from build123d import *

# Parameters (mm, degrees)
CROQUIS1_W              = 309
CROQUIS1_H              = 195
CROQUIS1_W_2            = 227
CROQUIS1_H_2            = 113
SALIENTE_EXTRUIR1_DEPTH = 15
CROQUIS2_R              = 2.75
CORTAR_EXTRUIR1_DEPTH   = 7.5


with BuildPart() as part:
    # Croquis1 → Saliente-Extruir1 (new body)
    with BuildSketch(Plane.YZ):
        with Locations((154.5, 97.5)):
            Rectangle(CROQUIS1_W, CROQUIS1_H)
        with Locations((154.5, 97.5)):
            Rectangle(CROQUIS1_W_2, CROQUIS1_H_2, mode=Mode.SUBTRACT)
    extrude(amount=SALIENTE_EXTRUIR1_DEPTH)

    # Croquis2 → Cortar-Extruir1 (cut)
    with BuildSketch(Plane.YZ.offset(15)):
        with BuildLine():
            ThreePointArc((66.75, 41), (64, 43.75), (61.25, 41))
            Line((61.25, 41), (66.75, 41))
        make_face()
        with BuildLine():
            Line((66.75, 41), (61.25, 41))
            ThreePointArc((61.25, 41), (64, 38.25), (66.75, 41))
        make_face()
        with Locations((116, 41)):
            Circle(CROQUIS2_R)
        with Locations((178, 41)):
            Circle(CROQUIS2_R)
    extrude(amount=-CORTAR_EXTRUIR1_DEPTH, mode=Mode.SUBTRACT)


solid = part.part
Can you work these out from the model? Positions are in its coordinate system, mm. A direction names the side the tool comes from. Coordinates: 2 decimals unless noted, no trailing zeros. Loops run counter-clockwise (first coordinate to the right, second up) from the corner with the lowest first, then second, coordinate; pieces in that order, holes last. Notation, with made-up numbers: M 78.25,-12 L 106.25,-12 A3 cw 106.25,-8 Z; hole C 19,-24 d6. An arc over 180 degrees is marked long. Return JSON: item names as keys, results as strings. Group by question number.
Item 1: Imagine slicing it at B-B (z = 126). Please give me the cut outline in (x, y).
Item 2: Imagine slicing it at A-A (x = 12.5). Please give me the cut outline in (y, z).
Item 3: I'm going to push a flat-ended pin straight in: pin 1 Ø0.8 at (y, z) = (177.5, 40) entering from +X. Where does the tip first touch, or does it pass through?
Item 4: On a 3-axis mill with a long thin cutter (end or side, diameter ignored), from which of +Z, -Z, +X, -X, +Y, -Y can I reach the whole of each face in a straight line? I mean faces 4 (the cylindrical face through (11.3, 177.94, 38.25)), 5 (the flat face through (15, 152, 34)), 6 (the flat face through (7, 268, 97)). Say none if no direction works.
Item 5: If I drill on L1, parallel to Y at x = 1.5, z = 49; L2, parallel to Z at x = 12.5, y = 156.5; L3, parallel to Z at x = 10.25, y = 115, over which ranges is the centre line in solid material (lowest first)? Write a range as from..to.
Item 6: Thinking about a two-plate mould opening in Y: for faces 1 (the flat face through (7, 309, 96)), 2 (the cylindrical face through (11.3, 115.94, 38.25)), 3 (the flat face through (7, 0, 96)), which applies, released by +Y, released by -Y, zero draft, split by the parting line, or undercut?
Verdict:
{
 "1": {"outline": "M 0,0 L 15,0 L 15,41 L 0,41 Z; M 0,268 L 15,268 L 15,309 L 0,309 Z"},
 "2": {"outline": "M 0,0 L 309,0 L 309,195 L 0,195 Z; hole M 41,41 L 61.25,41 A2.75 ccw 66.75,41 L 113.25,41 A2.75 ccw 118.75,41 L 175.25,41 A2.75 ccw 180.75,41 L 268,41 L 268,154 L 41,154 Z"},
 "3": {"pin 1": "stops at x = 7.5"},
 "4": {"face 4": "+X", "face 5": "+Z, -Z, +X, +Y, -Y", "face 6": "+X, -X"},
 "5": {"L1": "y = 0..41, 268..309", "L2": "z = 0..41, 154..195", "L3": "z = 0..38.44, 154..195"},
 "6": {"face 1": "released by +Y", "face 2": "undercut", "face 3": "released by -Y"}
}
